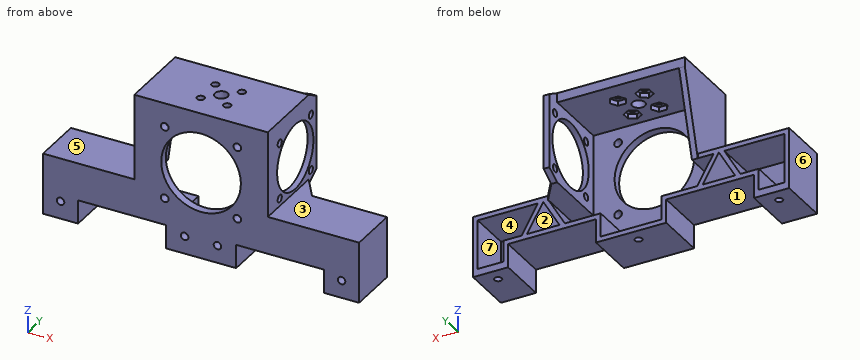
from build123d import *

# Parameters (mm, degrees)
SKETCH_2_R          = 1.6
SKETCH_2_R_2        = 17
SKETCH_2_R_3        = 1.65
EXTRUDE_2_DEPTH     = 3.5
EXTRUDE_3_DEPTH     = 18
EXTRUDE_4_DEPTH     = 10
CUT_EXTRUDE_5_DEPTH = 3
SKETCH_10_R         = 2.75
SKETCH_10_R_2       = 1.6
CUT_EXTRUDE_4_DEPTH = 5
EXTRUDE_5_DEPTH     = 18
SKETCH_14_R         = 1.55
CUT_EXTRUDE_6_DEPTH = 10
CUT_EXTRUDE_7_DEPTH = 2
EXTRUDE_6_DEPTH     = 2
EXTRUDE_7_DEPTH     = 2.5
SKETCH_21_R         = 1.6
SKETCH_21_R_2       = 14
CUT_EXTRUDE_8_DEPTH = 3


with BuildPart() as part:
    # 草图2 → 凸台-拉伸2 (new body)
    with BuildSketch(Plane(origin=(0, 0, 0), x_dir=(1, 0, 0), z_dir=(0, 1, 0))):
        Polygon((-39, 36.7), (-39, 62.8), (-24, 62.8), (-24, 52.7), (13.5, 52.7), (13.5, 62.8), (43.5, 62.8), (43.5, 52.7), (81, 52.7), (81, 62.8), (96, 62.8), (96, 36.7), (57, 36.7), (57, 0), (0, 0), (0, 36.7), align=None)
        with Locations(Location((-31.5, 55.3, 0), (0, 0, 270))):
            Circle(SKETCH_2_R, mode=Mode.SUBTRACT)
        with Locations(Location((88.5, 55.3, 0), (0, 0, 270))):
            Circle(SKETCH_2_R, mode=Mode.SUBTRACT)
        with Locations(Location((21.5, 55.3, 0), (0, 0, 270))):
            Circle(SKETCH_2_R, mode=Mode.SUBTRACT)
        with Locations(Location((35.5, 55.3, 0), (0, 0, 270))):
            Circle(SKETCH_2_R, mode=Mode.SUBTRACT)
        with Locations(Location((28.5, 25.7, 0), (0, 0, 270))):
            Circle(SKETCH_2_R_2, mode=Mode.SUBTRACT)
        with Locations(Location((44, 41.2, 0), (0, 0, 270))):
            Circle(SKETCH_2_R_3, mode=Mode.SUBTRACT)
        with Locations(Location((44, 10.2, 0), (0, 0, 270))):
            Circle(SKETCH_2_R_3, mode=Mode.SUBTRACT)
        with Locations(Location((13, 10.2, 0), (0, 0, 270))):
            Circle(SKETCH_2_R_3, mode=Mode.SUBTRACT)
        with Locations(Location((13, 41.2, 0), (0, 0, 270))):
            Circle(SKETCH_2_R_3, mode=Mode.SUBTRACT)
    extrude(amount=EXTRUDE_2_DEPTH)

    # 草图6 → 凸台-拉伸3 (add)
    with BuildSketch(Plane(origin=(0, 3.5, 0), x_dir=(1, 0, 0), z_dir=(0, 1, 0))):
        Polygon((13.5, 52.7), (-24, 52.7), (-24, 62.8), (-39, 62.8), (-39, 36.7), (0, 36.7), (0, 0), (57, 0), (57, 36.7), (96, 36.7), (96, 62.8), (81, 62.8), (81, 52.7), (43.5, 52.7), (43.5, 62.8), (13.5, 62.8), align=None)
        Polygon((15.5, 50.7), (-26, 50.7), (-26, 59.8), (-37, 59.8), (-37, 38.7), (2.5, 38.7), (2.5, 4), (54.5, 4), (54.5, 38.7), (94, 38.7), (94, 59.8), (83, 59.8), (83, 50.7), (41.5, 50.7), (41.5, 60.8), (15.5, 60.8), align=None, mode=Mode.SUBTRACT)
    extrude(amount=EXTRUDE_3_DEPTH)

    # 草图11 → 凸台-拉伸4 (add)
    with BuildSketch(Plane(origin=(0, 21.5, 0), x_dir=(1, 0, 0), z_dir=(0, 1, 0))):
        Polygon((2.5, 38.7), (2.5, 4), (54.5, 4), (54.5, 38.7), (57, 38.7), (57, 0), (0, 0), (0, 38.7), align=None)
    extrude(amount=EXTRUDE_4_DEPTH)

    # 草图12 → 切除-拉伸5 (cut)
    with BuildSketch(Plane.ZY):
        Polygon((-38.7, 21.5), (-4, 31.5), (-38.7, 31.5), align=None)
    extrude(amount=-CUT_EXTRUDE_5_DEPTH, mode=Mode.SUBTRACT)

    # 草图10 → 切除-拉伸4 (cut)
    with BuildSketch(Plane.XY):
        with Locations((28.5, 15.656854249)):
            Circle(SKETCH_10_R)
        with Locations((34.156854249, 21.313708499)):
            Circle(SKETCH_10_R_2)
        with Locations((34.156854249, 10)):
            Circle(SKETCH_10_R_2)
        with Locations((22.843145751, 10)):
            Circle(SKETCH_10_R_2)
        with Locations((22.843145751, 21.313708499)):
            Circle(SKETCH_10_R_2)
    extrude(amount=-CUT_EXTRUDE_4_DEPTH, mode=Mode.SUBTRACT)

    # 草图13 → 凸台-拉伸5 (add)
    with BuildSketch(Plane(origin=(0, 3.5, 0), x_dir=(1, 0, 0), z_dir=(0, 1, 0))):
        Polygon((-9, 38.7), (-15.92820323, 50.7), (-18.237604307, 50.7), (-11.309401077, 38.7), align=None)
        Polygon((-2.07179677, 50.7), (-9, 38.7), (-6.690598923, 38.7), (0.237604307, 50.7), align=None)
        Polygon((56.762395693, 50.7), (63.690598923, 38.7), (66, 38.7), (59.07179677, 50.7), align=None)
        Polygon((72.92820323, 50.7), (66, 38.7), (68.309401077, 38.7), (75.237604307, 50.7), align=None)
    extrude(amount=EXTRUDE_5_DEPTH)

    # 草图14 → 切除-拉伸6 (cut)
    with BuildSketch(Plane(origin=(0, 0, -62.8), x_dir=(-1, 0, 0), z_dir=(0, 0, -1))):
        with Locations((31.5, 15.656854249)):
            Circle(SKETCH_14_R)
        with Locations(Location((-88.5, 15.656854249, 0), (0, 0, 180))):
            Circle(SKETCH_14_R)
        with Locations((-28.5, 15.656854249)):
            Circle(SKETCH_14_R)
    extrude(amount=-CUT_EXTRUDE_6_DEPTH, mode=Mode.SUBTRACT)

    # 草图20 → 切除-拉伸7 (cut)
    with BuildSketch(Plane(origin=(0, 0, -4), x_dir=(-1, 0, 0), z_dir=(0, 0, -1))):
        Polygon((-25.843145751, 19.581657691), (-22.843145751, 17.849606884), (-19.843145751, 19.581657691), (-19.843145751, 23.045759307), (-22.843145751, 24.777810114), (-25.843145751, 23.045759307), align=None)
        Polygon((-32.424803442, 18.313708499), (-30.692752634, 21.313708499), (-32.424803442, 24.313708499), (-35.888905057, 24.313708499), (-37.620955865, 21.313708499), (-35.888905057, 18.313708499), align=None)
        Polygon((-24.575196558, 13), (-26.307247366, 10), (-24.575196558, 7), (-21.111094943, 7), (-19.379044135, 10), (-21.111094943, 13), align=None)
        Polygon((-31.156854249, 11.732050808), (-34.156854249, 13.464101615), (-37.156854249, 11.732050808), (-37.156854249, 8.267949192), (-34.156854249, 6.535898385), (-31.156854249, 8.267949192), align=None)
    extrude(amount=-CUT_EXTRUDE_7_DEPTH, mode=Mode.SUBTRACT)

    # 草图22 → 凸台-拉伸6 (add)
    with BuildSketch(Plane(origin=(0, 0, -38.7), x_dir=(-1, 0, 0), z_dir=(0, 0, -1))):
        Polygon((-57, 31.5), (-64.002075382, 21.5), (-57, 21.5), align=None)
    extrude(amount=-EXTRUDE_6_DEPTH)

    # 草图24 → 凸台-拉伸7 (add)
    with BuildSketch(Plane(origin=(57, 0, 0), x_dir=(0, 0, -1), z_dir=(1, 0, 0))):
        Polygon((0, 31.5), (3.464101615, 37.5), (35.235898385, 37.5), (38.7, 31.5), align=None)
    extrude(amount=-EXTRUDE_7_DEPTH)

    # 草图21 → 切除-拉伸8 (cut)
    with BuildSketch(Plane(origin=(57, 0, 0), x_dir=(0, 0, -1), z_dir=(1, 0, 0))):
        with Locations((9.5, 33.2)):
            Circle(SKETCH_21_R)
        with Locations((33.5, 33.2)):
            Circle(SKETCH_21_R)
        with Locations((33.5, 9.2)):
            Circle(SKETCH_21_R)
        with Locations((9.5, 9.2)):
            Circle(SKETCH_21_R)
        with Locations((21.5, 21.2)):
            Circle(SKETCH_21_R_2)
    extrude(amount=-CUT_EXTRUDE_8_DEPTH, mode=Mode.SUBTRACT)


solid = part.part
Here's how the part is built. I have some questions about the finished solid (model axes, mm). Face numbers are marked on the shaded views. A direction names the side the tool comes from. Coordinates: 2 decimals unless noted, no trailing zeros. Write each loop counter-clockwise with the first axis right and the second up, starting at its lowest first coordinate (ties: lowest second). Pieces come first, ordered by that corner, then holes.
Item 1: On a 3-axis mill with a long thin cutter (end or side, diameter ignored), from which of +Z, -Z, +X, -X, +Y, -Y can I reach the whole of each face in a straight line? I mean the marked faces 1, 2 and 3. Say none if no direction works.
Item 2: If we mould it in two halves opening along X, with no side actions, what happens to the marked faces 4, 5, 6 and 7? For each: +X half, -X half, draft (parallel to the pull), parting line (faces both ways), or undercut.
Item 3: I want a section at C-C on y = 27.5. Write out the boundary of the cut face in (x, z).
Item 4: Will these pins go through, and if not, where does the flat tip stop? pin 1 (1.5 mm diameter, centred on y = 30.5, z = -31.5, fed in from -X); pin 2 (1 mm diameter, centred on x = -12.5, z = -45, fed in from +Y); pin 3 (1.5 mm diameter, centred on y = 19, z = -12.5, fed in from -X).
Item 5: I want a section at B-B on x = 88.5. Write out the boundary of the cut face in (y, z).
Item 6: I want a section at A-A on z = -21.5. Write out the boundary of the cut face in (x, y), and give its area (3 significant figures).
Item 7: I want a section at D-D on x = 6. Write out the boundary of the cut face in (y, z).
Item 8: If I drill on line 1 (X direction, y = 4, z = -34); line 2 (Y direction, x = 56.05, z = -21.5); line 3 (Z direction, x = -5, y = 19), over which ranges is the centre line in solid material (lowest first)?
Findings below:
1. face 1: -Z, +Y, -Y
1. face 2: +Y
1. face 3: +Z, +X, +Y, -Y
2. face 4: undercut
2. face 5: draft
2. face 6: -X half
2. face 7: undercut
3. outline: (0, -17.88) - (2.5, -17.88) - (2.5, -4) - (54.5, -4) - (54.5, -9) - (57, -9) - (57, 0) - (0, 0) - close; (54.5, -38.7) - (59.8, -38.7) - (59.8, -36.7) - (57, -36.7) - (57, -34) - (54.5, -34) - close
4. pin 1: stops at x = 54.5
4. pin 2: stops at y = 21.5
4. pin 3: stops at x = 0
5. outline: (0, -62.8) - (14.11, -62.8) - (14.11, -59.8) - (3.5, -59.8) - (3.5, -56.9) - (0, -56.9) - close; (0, -53.7) - (3.5, -53.7) - (3.5, -38.7) - (21.5, -38.7) - (21.5, -36.7) - (0, -36.7) - close; (17.21, -62.8) - (21.5, -62.8) - (21.5, -59.8) - (17.21, -59.8) - close
6. outline: (0, 0) - (12.03, 0) - (12.03, 3.5) - (2.5, 3.5) - (2.5, 26.46) - (0, 26.46) - close; (44.97, 0) - (57, 0) - (57, 7.2) - (54.5, 7.2) - (54.5, 3.5) - (44.97, 3.5) - close; (54.5, 35.2) - (57, 35.2) - (57, 37.5) - (54.5, 37.5) - close
6. area: 157 mm2
7. outline: (0, -52.7) - (21.5, -52.7) - (21.5, -50.7) - (3.5, -50.7) - (3.5, -4) - (31.5, -4) - (31.5, 0) - (0, 0) - close
8. line 1: x = 0 to 2.5, 54.5 to 57
8. line 2: y = 0 to 7.2, 35.2 to 37.5
8. line 3: z = -52.7 to -50.7, -45.63 to -41.63, -38.7 to -36.7
